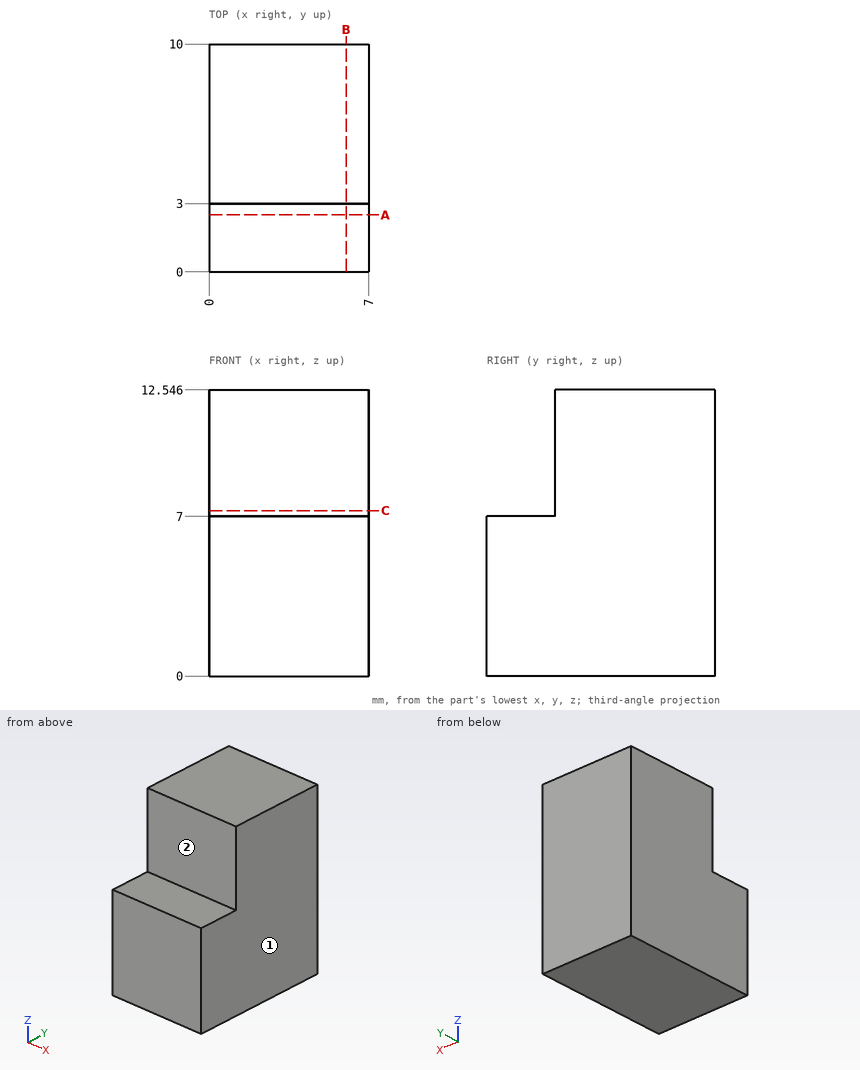
The figure shows three views and two pictorial views of one solid part (mm, origin at its lowest corner). Answer the questions. A direction names the side the tool comes from. Coordinates: 2 decimals unless noted, no trailing zeros. Loops run counter-clockwise (first coordinate to the right, second up) from the corner with the lowest first, then second, coordinate; pieces in that order, holes last. Notation, with made-up numbers: M -14.5,33.25 L 3.5,33.25 A26 ccw 3.5,72.25 Z; hole C 2.5,77 d7. An arc over 180 degrees is marked long. Answer as CSV lines item,"result". Start each with the question number.
(1) For the marked faces 1 and 2, determine the directions among +Z, -Z, +X, -X, +Y, -Y from which every point of the face is accessible in a straight line to the end or side of a thin tool.
(2) The part is cut by section C-C (z = 7.25). Give the vertices of the cut face in (x, y).
(3) Find the intervals of material crossed by L1, parallel to Z at x = 4, y = 2; L2, parallel to Y at x = 0.5, z = 9.5, in increasing order. Write a range as [from, to].
(4) The part is cut by section B-B (x = 6). Give the vertices of the cut face in (y, z) (1 decimal), and give its area (3 significant figures).
(5) The part is cut by section A-A (y = 2.5). Give the vertices of the cut face in (x, z), and give its area (3 significant figures).
Determined:
1,face 1,"+Z, -Z, +X, +Y, -Y"
1,face 2,"+Z, +X, -X, -Y"
2,outline,"M 0,3 L 7,3 L 7,10 L 0,10 Z"
3,L1,"[0, 7]"
3,L2,"[3, 10]"
4,outline,"M 0,0 L 10,0 L 10,12.5 L 3,12.5 L 3,7 L 0,7 Z"
4,area,"109 mm2"
5,outline,"M 0,0 L 7,0 L 7,7 L 0,7 Z"
5,area,"49.0 mm2"
